from build123d import *

# Parameters (mm, degrees)
SKETCH_W        = 39.5
SKETCH_H        = 20
PAD_DEPTH       = 3
SKETCH001_W     = 2
SKETCH001_H     = 10
PAD001_DEPTH    = 3
CHAMFER_SIZE    = 6.99
CHAMFER001_SIZE = 6.99


with BuildPart() as part:
    # Sketch → Pad (new body)
    with BuildSketch(Plane.XZ):
        with Locations((19.75, 10)):
            Rectangle(SKETCH_W, SKETCH_H)
    extrude(amount=PAD_DEPTH)

    # Sketch001 → Pad001 (new body)
    with BuildSketch(Plane(origin=(0, 0, 0), x_dir=(1, 0, 0), z_dir=(0, 0, -1))):
        with Locations((38.5, 5)):
            Rectangle(SKETCH001_W, SKETCH001_H)
        with Locations((1, 5)):
            Rectangle(SKETCH001_W, SKETCH001_H)
    extrude(amount=-PAD001_DEPTH)

    # Chamfer
    chamfer_edges = [part.edges().sort_by_distance(p)[0] for p in [
        (38.5, -3, 3),
    ]]
    chamfer(chamfer_edges, length=CHAMFER_SIZE)

    # Chamfer001
    chamfer001_edges = [part.edges().sort_by_distance(p)[0] for p in [
        (1, -3, 3),
    ]]
    chamfer(chamfer001_edges, length=CHAMFER001_SIZE)


solid = part.part
For this review, take the finished solid that the model builds, in its own axes (mm). A direction names the side the tool comes from. Round coordinates to 2 decimals unless told otherwise and drop trailing zeros. Order: outer loops, then holes, each group sorted by start corner. A loop starts at its lowest first (then second) coordinate and runs counter-clockwise, first axis right, second up. Notation, with made-up numbers: M 83.25,34 L 130.25,34 A31 ccw 130.25,72 Z; hole C 28.25,-1 d8. An arc over 180 degrees is marked long. Use a Markdown table: item, result. Add a question column.
Item 1: Add section B-B, the plane z = 4. Give the boundary of the cut face in (x, y), then the cut area to 3 significant figures.
Item 2: Insertion check: pin 1 (2 mm diameter, centred on x = 18.5, z = 6, fed in from -Y). The pin has a flat end and moves straight along its axis. Give the tip position at first contact, or say it passes through.
Item 3: Add section D-D, the plane z = 6.25. Give the boundary of the cut face in (x, y), then the cut area to 3 significant figures.
Item 4: Add section A-A, the plane y = -8.75. Give the boundary of the cut face in (x, z), then the cut area to 3 significant figures.
Item 5: To check wall thickness, follow line 1 along Y through (x, z) = (28, 6). State the ranges of the line that lie inside material, in increasing order.
Item 6: Mouldability with a two-part tool opening along X and no side actions: class faces 1 (the flat face through (39.5, -4, 8)), 2 (the flat face through (2, -6, 4)), 3 (the flat face through (15.1, -2.7, 0)) as released by +X, released by -X, zero draft, split by the parting line, or undercut.
Item 7: Tool access review of faces 4 (the flat face through (19, 0, 10)), 5 (the flat face through (37.5, -6, 4)): name each direction out of +Z, -Z, +X, -X, +Y, -Y from which nothing blocks a thin tool from reaching the whole face with its end or side.
Item 8: Add section C-C, the plane y = -3.75. Give the boundary of the cut face in (x, z), then the cut area to 3 significant figures.
Geometry results:
| question | item | result |
|---|---|---|
| 1 | outline | M 0,-8.99 L 2,-8.99 L 2,-3 L 37.5,-3 L 37.5,-8.99 L 39.5,-8.99 L 39.5,0 L 0,0 Z |
| 1 | area | 142 mm² |
| 2 | pin 1 | stops at y = -3 |
| 3 | outline | M 0,-6.74 L 2,-6.74 L 2,-3 L 37.5,-3 L 37.5,-6.74 L 39.5,-6.74 L 39.5,0 L 0,0 Z |
| 3 | area | 133 mm² |
| 4 | outline | M 0,0 L 2,0 L 2,4.24 L 0,4.24 Z; M 37.5,0 L 39.5,0 L 39.5,4.24 L 37.5,4.24 Z |
| 4 | area | 17.0 mm² |
| 5 | line 1 | y = -3 to 0 |
| 6 | face 1 | released by +X |
| 6 | face 2 | undercut |
| 6 | face 3 | zero draft |
| 7 | face 4 | +Z, -Z, +X, -X, +Y |
| 7 | face 5 | +Z, -Z, -Y |
| 8 | outline | M 0,0 L 2,0 L 2,9.24 L 0,9.24 Z; M 37.5,0 L 39.5,0 L 39.5,9.24 L 37.5,9.24 Z |
| 8 | area | 37.0 mm² |
